from build123d import *

# Parameters (mm, degrees)
SKETCH1_W           = 40
SKETCH1_H           = 3
SKETCH1_W_2         = 3
SKETCH1_H_2         = 90
BOSS_EXTRUDE1_DEPTH = 3


with BuildPart() as part:
    # Sketch1 → Boss-Extrude1 (new body)
    with BuildSketch(Plane.XY):
        with BuildLine():
            Line((97, 122), (-97, 122))
            ThreePointArc((-97, 122), (-99.121320344, 121.121320344), (-100, 119))
            Line((-100, 119), (-100, -119))
            ThreePointArc((-100, -119), (-99.121320344, -121.121320344), (-97, -122))
            Line((-97, -122), (97, -122))
            ThreePointArc((97, -122), (99.121320344, -121.121320344), (100, -119))
            Line((100, -119), (100, 119))
            ThreePointArc((100, 119), (99.121320344, 121.121320344), (97, 122))
        make_face()
        with Locations((-40, 123.5)):
            Rectangle(SKETCH1_W, SKETCH1_H)
        with Locations((40, 123.5)):
            Rectangle(SKETCH1_W, SKETCH1_H)
        with Locations((-101.5, 0)):
            Rectangle(SKETCH1_W_2, SKETCH1_H_2)
        with Locations((101.5, 0)):
            Rectangle(SKETCH1_W_2, SKETCH1_H_2)
        with Locations((40, -123.5)):
            Rectangle(SKETCH1_W, SKETCH1_H)
        with Locations((-40, -123.5)):
            Rectangle(SKETCH1_W, SKETCH1_H)
    extrude(amount=BOSS_EXTRUDE1_DEPTH)


solid = part.part
Design review of the part built by this model. Coordinates are the model's own, in mm. Coordinates: 2 decimals unless noted, no trailing zeros. Order: outer loops, then holes, each group sorted by start corner. A loop starts at its lowest first (then second) coordinate and runs counter-clockwise, first axis right, second up.
Item 1: Take a section at B-B, the plane y = -74.5. Write out the cut boundary in (x, z), then the cut area to 3 significant figures.
Item 2: Take a section at C-C, the plane x = 78.5. Write out the cut boundary in (y, z).
Item 3: For pin 1 Ø1 at (y, z) = (-71.5, 2.5) entering from +X; pin 2 Ø1.5 at (y, z) = (124, 1.5) entering from +X; pin 3 Ø1.5 at (x, z) = (78.5, 1.5) entering from -Y; pin 4 Ø1 at (x, y) = (-13.5, 87) entering from -Z, all flat-tipped, find the tip position at first contact; note any pin that passes through.
Item 4: For line 1 (X direction, y = -77.5, z = 1.5); line 2 (Y direction, x = -80.5, z = 2.1), list the stretches that pass through material, from the lowest coordinate up.
The answers:
1. outline: (-100, 0) - (100, 0) - (100, 3) - (-100, 3) - close
1. area: 600 mm2
2. outline: (-122, 0) - (122, 0) - (122, 3) - (-122, 3) - close
3. pin 1: stops at x = 100
3. pin 2: stops at x = 60
3. pin 3: stops at y = -122
3. pin 4: stops at z = 0
4. line 1: x = -100 to 100
4. line 2: y = -122 to 122
